Design review of the part built by this model. Coordinates are the model's own, in mm. Face numbers are marked on the shaded views. A direction names the side the tool comes from. Coordinates: 2 decimals unless noted, no trailing zeros. Write each loop counter-clockwise with the first axis right and the second up, starting at its lowest first coordinate (ties: lowest second). Pieces come first, ordered by that corner, then holes. Notation, with made-up numbers: (74, 12) - (87, 12) arc R29 cw to (87, 45) - close; hole circle Ø9 at (67, -34.5). An arc over 180 degrees is marked (long way). One line per item, written item: value.
from build123d import *

# Parameters (mm, degrees)
F0_W     = 16
F0_H     = 16
F0_R     = 3.25
F1_DEPTH = 10
F2_DEPTH = 6
F3_SIZE  = 1.9


with BuildPart() as f1:
    # F0 (on Top) → F1 (new body)
    with BuildSketch(Plane.XY):
        Rectangle(F0_W, F0_H)
        Polygon((-6.004443, 0), (-3.002221, 5.2), (3.002221, 5.2), (6.004443, 0), (3.002221, -5.2), (-3.002221, -5.2), align=None, mode=Mode.SUBTRACT)
        Polygon((3.002221, 5.2), (-3.002221, 5.2), (-6.004443, 0), (-3.002221, -5.2), (3.002221, -5.2), (6.004443, 0), align=None)
        Circle(F0_R, mode=Mode.SUBTRACT)
    extrude(amount=F1_DEPTH)

    # F0 (on Top) → F2 (cut)
    with BuildSketch(Plane.XY):
        Polygon((3.002221, 5.2), (-3.002221, 5.2), (-6.004443, 0), (-3.002221, -5.2), (3.002221, -5.2), (6.004443, 0), align=None)
        Circle(F0_R, mode=Mode.SUBTRACT)
    extrude(amount=F2_DEPTH, mode=Mode.SUBTRACT)

    # F3
    f3_edges = [f1.edges().sort_by_distance(p)[0] for p in [
        (0, 8, 0),
        (0, -8, 0),
        (0, 8, 10),
        (0, -8, 10),
    ]]
    chamfer(f3_edges, length=F3_SIZE)


solid = f1.part
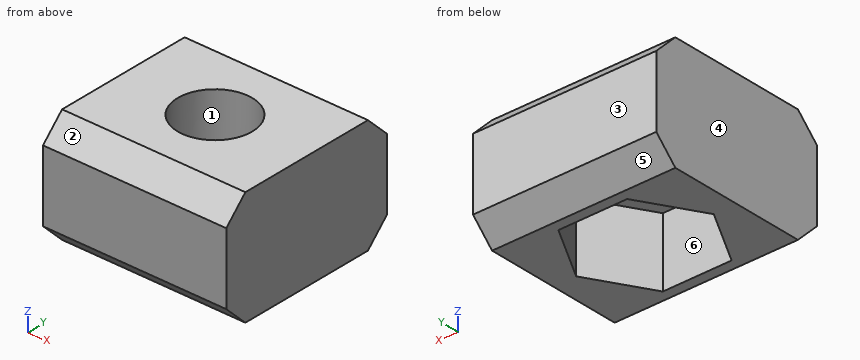
1. Consider section A-A, the plane z = 4. Write out the cut boundary in (x, y).
Answer block:
outline: (-8, -8) - (8, -8) - (8, 8) - (-8, 8) - close; hole (-6, 0) - (-3, -5.2) - (3, -5.2) - (6, 0) - (3, 5.2) - (-3, 5.2) - close
2. For the marked faces 5 and 6, list the 3-axis set-ups (+Z, -Z, +X, -X, +Y, -Y) from which the entire face can be reached by the end or side of a thin tool; tool diameter is ignored.
Answer block:
face 5: -Z, +X, -X, +Y
face 6: -Z
3. Mouldability with a two-part tool opening along Y and no side actions: class the marked faces 1, 2, 3 and 4 as released by +Y, released by -Y, zero draft, split by the parting line, or undercut.
Answer block:
face 1: undercut
face 2: released by -Y
face 3: released by +Y
face 4: zero draft
4. Consider section D-D, the plane x = 6.75. Write out the cut boundary in (y, z).
Answer block:
outline: (-8, 1.9) - (-6.1, 0) - (6.1, 0) - (8, 1.9) - (8, 8.1) - (6.1, 10) - (-6.1, 10) - (-8, 8.1) - close
5. Insertion check: pin 1 Ø1.8 at (x, z) = (-1, 1.5) entering from -Y; pin 2 Ø5 at (x, y) = (-1.5, -0.5) entering from -Z. Each pin has a flat end and moves straight along its axis. Give the tip position at first contact, or say it passes through.
Answer block:
pin 1: stops at y = -8
pin 2: stops at z = 6
6. Consider section C-C, the plane y = -3. Write out the cut boundary in (x, z), then the cut area to 3 significant figures.
Answer block:
outline: (-8, 0) - (-4.27, 0) - (-4.27, 6) - (-1.25, 6) - (-1.25, 10) - (-8, 10) - close; (1.25, 6) - (4.27, 6) - (4.27, 0) - (8, 0) - (8, 10) - (1.25, 10) - close
area: 98.7 mm^2
7. Consider section B-B, the plane x = 0. Write out the cut boundary in (y, z), then the cut area to 3 significant figures.
Answer block:
outline: (-8, 1.9) - (-6.1, 0) - (-5.2, 0) - (-5.2, 6) - (-3.25, 6) - (-3.25, 10) - (-6.1, 10) - (-8, 8.1) - close; (3.25, 6) - (5.2, 6) - (5.2, 0) - (6.1, 0) - (8, 1.9) - (8, 8.1) - (6.1, 10) - (3.25, 10) - close
area: 64.4 mm^2
8. Wall thickness on line 1 along Y through (x, z) = (0, 6.25); line 2 along Z through (x, y) = (-1.75, 3); line 3 along Y through (x, z) = (0, 8.4): over which ranges is each line inside the solid? List them lowest first.
Answer block:
line 1: y = -8 to -3.25, 3.25 to 8
line 2: z = 6 to 10
line 3: y = -7.7 to -3.25, 3.25 to 7.7
